The model under review builds one solid part; all positions refer to its coordinate system, in mm. Face numbers are marked on the shaded views. A direction names the side the tool comes from. Coordinates: 2 decimals unless noted, no trailing zeros. Write each loop counter-clockwise with the first axis right and the second up, starting at its lowest first coordinate (ties: lowest second). Pieces come first, ordered by that corner, then holes. Notation, with made-up numbers: (55.25, 32) - (92.25, 32) arc R22 cw to (92.25, 43) - close; hole circle Ø6 at (-36.75, -31.75). An arc over 180 degrees is marked (long way). Use one line per item in the form item = value. Start each with the question number.
Autodesk Inventor part; units mm, degrees
ref_plane "YZ Plane" through (0, 0, 0) normal (1, 0, 0) x (0, 1, 0)
ref_plane "XZ Plane" through (0, 0, 0) normal (0, 1, 0) x (-1, 0, 0)
ref_plane "XY Plane" through (0, 0, 0) normal (0, 0, 1) x (1, 0, 0)
sketch "Sketch1" plane through (0, 0, 0) normal (0, 0, 1) x (1, 0, 0)
  line L0 (0, 0) -> (45, 0)
  line L1 (45, 0) -> (45, 8)
  line L2 (45, 8) -> (0, 8)
  line L3 (0, 8) -> (0, 0)
  circle A0 centre (5, 4) radius 1
  circle A1 centre (40, 4) radius 1
  point P0 (0, 4)
  dimension "d0" = 45
  dimension "d1" = 8
  dimension "d2" = 2
  dimension "d3" = 2
  dimension "d4" = 5
  dimension "d5" = 5
extrude "Extrusion1" add sketch "Sketch1" along normal blind 3
fillet "Fillet1" radius 2 4 edges at (0, 8, 1.5) (45, 8, 1.5) (45, 0, 1.5) (0, 0, 1.5)
chamfer "Chamfer1" distance 2 angle 45 2 edges at (4, 4, 3) (39, 4, 0)
sketch "Sketch2" plane through (0, 0, 0) normal (0, 0, -1) x (-1, 0, 0)
  circle A0 centre (-5, 4) radius 1
  circle A1 centre (-5, 4) radius 4
  point P0 (0, 0)
  dimension "d12" = 8
extrude "Extrusion2" add sketch "Sketch2" along normal blind 4
equation "\"d5\" = d4"
properties part number "arm"
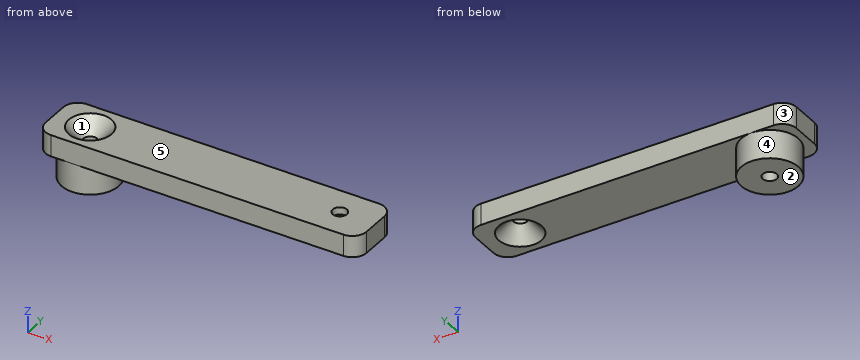
1. Take a section at A-A (x = 40). State the section outline as (y, z) points, plus the area to 3 significant figures.
2. For the marked faces 4 and 5, list the 3-axis set-ups (+Z, -Z, +X, -X, +Y, -Y) from which the entire face can be reached by the end or side of a thin tool; tool diameter is ignored.
3. Take a section at D-D (x = 28). State the section outline as (y, z) points, plus the area to 3 significant figures.
4. For P1, Ø2.5, axis at x = 40, y = 4, coming from the -Z side; P2, Ø2.5, axis at x = 5, y = 4, coming from the +Z side; P3, Ø2.5, axis at x = 18.5, y = 5, coming from the -Z side, all flat-tipped, find the tip position at first contact; note any pin that passes through.
5. Take a section at C-C (z = 0.5). State the section outline as (x, y) points.
6. Take a section at B-B (y = 4). State the section outline as (x, z) points.
7. The part is to be moulded in two halves that separate along X. For the marked faces 1, 2 and 3, say which applies: released by +X, released by -X, zero draft, split by the parting line, or undercut.
8. For L1, parallel to X at y = 4, z = -2.1; L2, parallel to Y at x = 5, z = -2.8; L3, parallel to X at y = 4.5, z = 2, list the stretches that pass through material, from the lowest coordinate up.
Returned:
q1.outline = (0, 0) - (1, 0) - (3, 2) - (3, 3) - (0, 3) - close; (5, 2) - (7, 0) - (8, 0) - (8, 3) - (5, 3) - close
q1.area = 14.0 mm²
q2.face_4 = -Z
q2.face_5 = +Z, +X, -X, +Y, -Y
q3.outline = (0, 0) - (8, 0) - (8, 3) - (0, 3) - close
q3.area = 24.0 mm²
q4.P1 = 1.75
q4.P2 = 1.25
q4.P3 = 0
q5.outline = (0, 2) arc R2 ccw to (2, 0) - (43, 0) arc R2 ccw to (45, 2) - (45, 6) arc R2 ccw to (43, 8) - (2, 8) arc R2 ccw to (0, 6) - close; hole circle Ø2 at (5, 4); hole circle Ø5 at (40, 4)
q6.outline = (0, 0) - (1, 0) - (1, -4) - (4, -4) - (4, 1) - (2, 3) - (0, 3) - close; (6, -4) - (9, -4) - (9, 0) - (37, 0) - (39, 2) - (39, 3) - (8, 3) - (6, 1) - close; (41, 2) - (43, 0) - (45, 0) - (45, 3) - (41, 3) - close
q7.face_1 = undercut
q7.face_2 = zero draft
q7.face_3 = released by -X
q8.L1 = 1 to 4, 6 to 9
q8.L2 = 0 to 3, 5 to 8
q8.L3 = 0 to 3.06, 6.94 to 39.13, 40.87 to 45
